The model under review builds one solid part; all positions refer to its coordinate system, in mm. A direction names the side the tool comes from. Coordinates: 2 decimals unless noted, no trailing zeros. Loops run counter-clockwise (first coordinate to the right, second up) from the corner with the lowest first, then second, coordinate; pieces in that order, holes last. Notation, with made-up numbers: (22.25, 38.25) - (30.25, 38.25) arc R13 ccw to (30.25, 58.25) - close; hole circle Ø11 at (44, 32.25). An arc over 180 degrees is marked (long way). One line per item, written item: value. Start each with the question number.
1. For faces 1 (the face through (-31.244, 2.435, 67.281)), 2 (the face through (-3, -14.12, 20.59)), list the 3-axis set-ups (+Z, -Z, +X, -X, +Y, -Y) from which the entire face can be reached by the end or side of a thin tool; tool diameter is ignored.
2. We need section B-B, the plane z = 47.5. Give the boundary of the cut face in (x, y) (1 decimal), then the cut area to 3 significant figures.
3. To check wall thickness, follow line 1 (Y direction, x = 4.5, z = 53); line 2 (X direction, y = 3.5, z = 94); line 3 (X direction, y = 5.5, z = 92.5). State the ranges of each line that lie inside material, in increasing order.
4. We need section A-A, the plane y = 4.5. Give the boundary of the cut face in (x, z).
5. We need section C-C, the plane y = -2. Give the boundary of the cut face in (x, z), then the cut area to 3 significant figures.
6. We need section D-D, the plane x = 22.5. Give the boundary of the cut face in (y, z).
7. Insertion check: P1, Ø2, axis at x = 2.5, z = 86, coming from the +Y side. The pin has a flat end and moves straight along its axis. Give the tip position at first contact, or say it passes through.
8. Mouldability with a two-part tool opening along X and no side actions: class faces 3 (the face through (-7, -12.986, 67)), 4 (the face through (38.1, 0, 68)), 5 (the face through (36, 17.431, 68)) as +X half, -X half, draft (parallel to the pull), parting line (faces both ways), or undercut.
from build123d import *

# Parameters (mm, degrees)
BOSS_EXTRUDE1_DEPTH     = 136.398
CUT_EXTRUDE1_DEPTH      = 18.43075
CUT_EXTRUDE1_DEPTH_BACK = 18.43075


with BuildPart() as part:
    # Sketch1 → Boss-Extrude1 (new body)
    with BuildSketch(Plane.XY):
        Polygon((-28.7655, -12.98575), (28.7655, -12.98575), (33.655, 17.43075), (38.1, 17.43075), (38.1, -17.43075), (-38.1, -17.43075), (-38.1, 17.43075), (-33.655, 17.43075), align=None)
    extrude(amount=BOSS_EXTRUDE1_DEPTH)

    # Sketch2 → Cut-Extrude1 (cut, two sides)
    with BuildSketch(Plane(origin=(0, 0, 0), x_dir=(1, 0, 0), z_dir=(0, 1, 0))) as cut_extrude1_sk:
        Polygon((-38.1, 0), (38.1, -44.704), (38.1, 0), align=None)
        Polygon((-38.1, -136.398), (38.1, -91.694), (38.1, -136.398), align=None)
    extrude(amount=CUT_EXTRUDE1_DEPTH, mode=Mode.SUBTRACT)
    extrude(cut_extrude1_sk.sketch, amount=-CUT_EXTRUDE1_DEPTH_BACK, mode=Mode.SUBTRACT)


solid = part.part
Findings below:
1. face 1: +Z, -Z, +Y
1. face 2: -Z, +X, +Y, -Y
2. outline: (-38.1, -17.4) - (38.1, -17.4) - (38.1, 17.4) - (33.7, 17.4) - (28.8, -13) - (-28.8, -13) - (-33.7, 17.4) - (-38.1, 17.4) - close
2. area: 758 mm2
3. line 1: -17.43 to -12.99
3. line 2: -38.1 to -31.42, 31.42 to 34.17
3. line 3: -38.1 to -31.74, 31.74 to 36.73
4. outline: (-38.1, 0) - (-31.58, 3.83) - (-31.58, 132.57) - (-38.1, 136.4) - close; (31.58, 40.88) - (38.1, 44.7) - (38.1, 91.69) - (31.58, 95.52) - close
5. outline: (-38.1, 0) - (-30.53, 4.44) - (-30.53, 131.96) - (-38.1, 136.4) - close; (30.53, 40.26) - (38.1, 44.7) - (38.1, 91.69) - (30.53, 96.13) - close
5. area: 1,390 mm2
6. outline: (-17.43, 35.55) - (-12.99, 35.55) - (-12.99, 100.85) - (-17.43, 100.85) - close
7. P1: y = -12.99
8. face 3: undercut
8. face 4: +X half
8. face 5: draft
